```python
from build123d import *

# Parameters (mm, degrees)
SKETCH1_W            = 58.2
SKETCH1_H            = 40
BOSS_EXTRUDE1_DEPTH  = 27
SKETCH2_R            = 3
BOSS_EXTRUDE2_DEPTH  = 2
SKETCH3_R            = 2
CUT_EXTRUDE1_DEPTH   = 31
SKETCH4_R            = 3
BOSS_EXTRUDE3_DEPTH  = 2
SKETCH5_R            = 2
CUT_EXTRUDE2_DEPTH   = 31
SKETCH6_R            = 3
BOSS_EXTRUDE4_DEPTH  = 2
SKETCH7_R            = 2
CUT_EXTRUDE3_DEPTH   = 31
SKETCH8_R            = 3
BOSS_EXTRUDE5_DEPTH  = 2
SKETCH9_R            = 2
CUT_EXTRUDE4_DEPTH   = 31
SKETCH10_R           = 8
BOSS_EXTRUDE6_DEPTH  = 4.5
SKETCH11_R           = 4
CUT_EXTRUDE5_DEPTH   = 36
BOSS_EXTRUDE7_START  = 2
SKETCH12_R           = 3
BOSS_EXTRUDE7_DEPTH  = 2
BOSS_EXTRUDE8_START  = 2
SKETCH13_R           = 3
BOSS_EXTRUDE8_DEPTH  = 2
BOSS_EXTRUDE9_START  = 4.5
SKETCH15_R           = 8
BOSS_EXTRUDE9_DEPTH  = 4.5
SKETCH18_R           = 2
CUT_EXTRUDE11_DEPTH  = 78.32716211
SKETCH19_R           = 4
CUT_EXTRUDE12_DEPTH  = 78.32716211
SKETCH20_R           = 2
CUT_EXTRUDE13_DEPTH  = 78.32716211
SKETCH24_R           = 3
BOSS_EXTRUDE11_DEPTH = 2
SKETCH25_R           = 3
BOSS_EXTRUDE12_DEPTH = 2
BOSS_EXTRUDE13_START = 2
SKETCH26_R           = 3
BOSS_EXTRUDE13_DEPTH = 2
BOSS_EXTRUDE14_START = 2
SKETCH27_R           = 3
BOSS_EXTRUDE14_DEPTH = 2
FILLET5_R            = 1.5
FILLET6_R            = 1.5


with BuildPart() as part:
    # Sketch1 → Boss-Extrude1 (new body)
    with BuildSketch(Plane(origin=(0, 0, 0), x_dir=(1, 0, 0), z_dir=(0, 1, 0))):
        with Locations((-29.1, 20)):
            Rectangle(SKETCH1_W, SKETCH1_H)
    extrude(amount=BOSS_EXTRUDE1_DEPTH)

    # Sketch2 → Boss-Extrude2 (add)
    with BuildSketch(Plane(origin=(0, 27, 0), x_dir=(1, 0, 0), z_dir=(0, 1, 0))):
        with Locations(Location((-49.1, 34, 0), (0, 0, 270))):
            Circle(SKETCH2_R)
    extrude(amount=BOSS_EXTRUDE2_DEPTH)

    # Sketch3 → Cut-Extrude1 (cut)
    with BuildSketch(Plane(origin=(0, 29, 0), x_dir=(1, 0, 0), z_dir=(0, 1, 0))):
        with Locations(Location((-49.1, 34, 0), (0, 0, 270))):
            Circle(SKETCH3_R)
    extrude(amount=-CUT_EXTRUDE1_DEPTH, mode=Mode.SUBTRACT)

    # Sketch4 → Boss-Extrude3 (add)
    with BuildSketch(Plane(origin=(0, 27, 0), x_dir=(1, 0, 0), z_dir=(0, 1, 0))):
        with Locations(Location((-9.1, 34, 0), (0, 0, 270))):
            Circle(SKETCH4_R)
    extrude(amount=BOSS_EXTRUDE3_DEPTH)

    # Sketch5 → Cut-Extrude2 (cut)
    with BuildSketch(Plane(origin=(0, 29, 0), x_dir=(1, 0, 0), z_dir=(0, 1, 0))):
        with Locations(Location((-9.1, 34, 0), (0, 0, 270))):
            Circle(SKETCH5_R)
    extrude(amount=-CUT_EXTRUDE2_DEPTH, mode=Mode.SUBTRACT)

    # Sketch6 → Boss-Extrude4 (add)
    with BuildSketch(Plane(origin=(0, 27, 0), x_dir=(1, 0, 0), z_dir=(0, 1, 0))):
        with Locations(Location((-49.1, 6, 0), (0, 0, 270))):
            Circle(SKETCH6_R)
    extrude(amount=BOSS_EXTRUDE4_DEPTH)

    # Sketch7 → Cut-Extrude3 (cut)
    with BuildSketch(Plane(origin=(0, 29, 0), x_dir=(1, 0, 0), z_dir=(0, 1, 0))):
        with Locations(Location((-49.1, 6, 0), (0, 0, 270))):
            Circle(SKETCH7_R)
    extrude(amount=-CUT_EXTRUDE3_DEPTH, mode=Mode.SUBTRACT)

    # Sketch8 → Boss-Extrude5 (add)
    with BuildSketch(Plane(origin=(0, 27, 0), x_dir=(1, 0, 0), z_dir=(0, 1, 0))):
        with Locations(Location((-9.1, 6, 0), (0, 0, 270))):
            Circle(SKETCH8_R)
    extrude(amount=BOSS_EXTRUDE5_DEPTH)

    # Sketch9 → Cut-Extrude4 (cut)
    with BuildSketch(Plane(origin=(0, 29, 0), x_dir=(1, 0, 0), z_dir=(0, 1, 0))):
        with Locations(Location((-9.1, 6, 0), (0, 0, 270))):
            Circle(SKETCH9_R)
    extrude(amount=-CUT_EXTRUDE4_DEPTH, mode=Mode.SUBTRACT)

    # Sketch10 → Boss-Extrude6 (add)
    with BuildSketch(Plane(origin=(0, 27, 0), x_dir=(1, 0, 0), z_dir=(0, 1, 0))):
        with Locations(Location((-20.5, 20, 0), (0, 0, 270))):
            Circle(SKETCH10_R)
    extrude(amount=BOSS_EXTRUDE6_DEPTH)

    # Sketch11 → Cut-Extrude5 (cut)
    with BuildSketch(Plane(origin=(0, 31.5, 0), x_dir=(1, 0, 0), z_dir=(0, 1, 0))):
        with Locations(Location((-20.5, 20, 0), (0, 0, 270))):
            Circle(SKETCH11_R)
    extrude(amount=-CUT_EXTRUDE5_DEPTH, mode=Mode.SUBTRACT)

    # Sketch12 → Boss-Extrude7 (add)
    with BuildSketch(Plane.XZ.offset(BOSS_EXTRUDE7_START)):
        with Locations(Location((-49.1, -6, 0), (0, 0, 90))):
            Circle(SKETCH12_R)
    extrude(amount=-BOSS_EXTRUDE7_DEPTH)

    # Sketch13 → Boss-Extrude8 (add)
    with BuildSketch(Plane.XZ.offset(BOSS_EXTRUDE8_START)):
        with Locations(Location((-49.1, -34, 0), (0, 0, 90))):
            Circle(SKETCH13_R)
        with Locations(Location((-9.1, -6, 0), (0, 0, 90))):
            Circle(SKETCH13_R)
        with Locations(Location((-9.1, -34, 0), (0, 0, 90))):
            Circle(SKETCH13_R)
    extrude(amount=-BOSS_EXTRUDE8_DEPTH)

    # Sketch15 → Boss-Extrude9 (add)
    with BuildSketch(Plane.XZ.offset(BOSS_EXTRUDE9_START)):
        with Locations(Location((-20.5, -20, 0), (0, 0, 90))):
            Circle(SKETCH15_R)
    extrude(amount=-BOSS_EXTRUDE9_DEPTH)

    # Sketch18 → Cut-Extrude11 (cut, through all)
    with BuildSketch(Plane(origin=(0, 0, 0), x_dir=(1, 0, 0), z_dir=(0, 1, 0))):
        with Locations(Location((-9.1, 6, 0), (0, 0, 270))):
            Circle(SKETCH18_R)
    extrude(amount=-CUT_EXTRUDE11_DEPTH, mode=Mode.SUBTRACT)

    # Sketch19 → Cut-Extrude12 (cut, through all)
    with BuildSketch(Plane(origin=(0, 0, 0), x_dir=(1, 0, 0), z_dir=(0, 1, 0))):
        with Locations(Location((-20.5, 20, 0), (0, 0, 270))):
            Circle(SKETCH19_R)
    extrude(amount=-CUT_EXTRUDE12_DEPTH, mode=Mode.SUBTRACT)

    # Sketch20 → Cut-Extrude13 (cut, through all)
    with BuildSketch(Plane(origin=(0, 0, 0), x_dir=(1, 0, 0), z_dir=(0, 1, 0))):
        with Locations(Location((-49.1, 34, 0), (0, 0, 270))):
            Circle(SKETCH20_R)
        with Locations(Location((-49.1, 6, 0), (0, 0, 270))):
            Circle(SKETCH20_R)
        with Locations(Location((-9.1, 34, 0), (0, 0, 270))):
            Circle(SKETCH20_R)
    extrude(amount=-CUT_EXTRUDE13_DEPTH, mode=Mode.SUBTRACT)

    # Sketch24 → Boss-Extrude11 (add)
    with BuildSketch(Plane(origin=(0, 27, 0), x_dir=(1, 0, 0), z_dir=(0, 1, 0))):
        with Locations(Location((-36.2, 15, 0), (0, 0, 270))):
            Circle(SKETCH24_R)
    extrude(amount=BOSS_EXTRUDE11_DEPTH)

    # Sketch25 → Boss-Extrude12 (add)
    with BuildSketch(Plane(origin=(0, 27, 0), x_dir=(1, 0, 0), z_dir=(0, 1, 0))):
        with Locations(Location((-36.2, 25, 0), (0, 0, 270))):
            Circle(SKETCH25_R)
    extrude(amount=BOSS_EXTRUDE12_DEPTH)

    # Sketch26 → Boss-Extrude13 (add)
    with BuildSketch(Plane.XZ.offset(BOSS_EXTRUDE13_START)):
        with Locations(Location((-36.2, -15, 0), (0, 0, 90))):
            Circle(SKETCH26_R)
    extrude(amount=-BOSS_EXTRUDE13_DEPTH)

    # Sketch27 → Boss-Extrude14 (add)
    with BuildSketch(Plane.XZ.offset(BOSS_EXTRUDE14_START)):
        with Locations(Location((-36.2, -25, 0), (0, 0, 90))):
            Circle(SKETCH27_R)
    extrude(amount=-BOSS_EXTRUDE14_DEPTH)

    # Fillet5
    fillet5_edges = [part.edges().sort_by_distance(p)[0] for p in [
        (-58.2, 27, -20),
        (-29.1, 27, 0),
        (0, 27, -20),
        (-29.1, 0, 0),
        (-58.2, 0, -20),
        (-29.1, 0, -40),
        (0, 0, -20),
        (0, 13.5, 0),
        (-58.2, 13.5, 0),
        (-58.2, 13.5, -40),
        (-29.1, 27, -40),
    ]]
    fillet(fillet5_edges, radius=FILLET5_R)

    # Fillet6
    # the kernel refuses this fillet: 1.5 mm, written as the material it takes off along each edge
    with BuildSketch(Plane(origin=(-1.5, 1.5, -38.5), x_dir=(0, 0, -1), z_dir=(1, 0, 0))) as fillet6_piece_1_section:
        Polygon((0, 0), (FILLET6_R, 0), (FILLET6_R, -FILLET6_R), (0, -FILLET6_R), align=None)
    fillet6_piece_1 = extrude(amount=FILLET6_R, mode=Mode.PRIVATE)
    fillet6_piece_1 = fillet6_piece_1 - Plane(origin=(-1.5, 1.5, -38.5), x_dir=(0, 0.7071067811865475, 0.7071067811865475), z_dir=(1, 0, 0)) * Sphere(FILLET6_R, mode=Mode.PRIVATE)
    add(fillet6_piece_1, mode=Mode.SUBTRACT)
    with BuildSketch(Plane(origin=(-1.5, 25.5, -38.5), x_dir=(0, 0, -1), z_dir=(1, 0, 0))) as fillet6_piece_2_section:
        Polygon((0, 0), (FILLET6_R, 0), (FILLET6_R, FILLET6_R), (0, FILLET6_R), align=None)
    fillet6_piece_2 = extrude(amount=FILLET6_R, mode=Mode.PRIVATE)
    fillet6_piece_2 = fillet6_piece_2 - Plane(origin=(-1.5, 25.5, -38.5), x_dir=(0, -0.7071067811865475, 0.7071067811865475), z_dir=(1, 0, 0)) * Sphere(FILLET6_R, mode=Mode.PRIVATE)
    add(fillet6_piece_2, mode=Mode.SUBTRACT)
    with BuildSketch(Plane(origin=(0, 1.5, -40), x_dir=(0, 0, 1), z_dir=(0, 1, 0))) as fillet6_piece_3:
        with BuildLine():
            CenterArc((FILLET6_R, -FILLET6_R), FILLET6_R, 90, 90)
            Line((0, -FILLET6_R), (0, 0))
            Line((0, 0), (FILLET6_R, 0))
        make_face()
    extrude(amount=24, mode=Mode.SUBTRACT)


solid = part.part
```
Source: CAD feature listing. Evaluate the final solid. Frame: model axes, mm. A direction names the side the tool comes from. Round coordinates to 2 decimals unless told otherwise and drop trailing zeros. Loops run counter-clockwise (first coordinate to the right, second up) from the corner with the lowest first, then second, coordinate; pieces in that order, holes last.
1. Mould query, pull axis Z, two halves, no side actions, for faces 1 (the flat face through (-48, -2, -32)), 2 (the cylindrical face through (-49, -1, -37)), 3 (the cylindrical face through (-46.438, -1.014, -4.616)), 4 (the cylindrical face through (-57.77, 13.67, -0.45)). Classes: released by +Z, released by -Z, zero draft, split by the parting line, or undercut.
2. Section query C-C on x = -20.5. Output: boundary loops of the cut face in (y, z), and give its area (3 significant figures).
3. Section query D-D on y = 19.5. Output: boundary loops of the cut face in (x, z), and give its area (3 significant figures).
4. Contact query for flat-ended pins moving along their axis: pin 1 (5 mm diameter, centred on x = -35.5, z = -16, fed in from +Y); pin 2 (5 mm diameter, centred on x = -47.5, z = -34, fed in from -Y); pin 3 (2 mm diameter, centred on x = -7, z = -17.5, fed in from +Y). Output: stop coordinate, or through.
5. Ray query, L1, parallel to Z at x = -49, y = 13; L2, parallel to X at y = 11.5, z = -34; L3, parallel to X at y = 18, z = -20. Return the intervals inside material, ascending.
6. Access query for faces 5 (the cylindrical face through (-38.23, -1.01, -27.21)), 6 (the flat face through (-36, -2, -25)), 7 (the cylindrical face through (-8.2, 27.99, -3.14)). Directions: +Z, -Z, +X, -X, +Y, -Y. A direction counts if a zero-diameter tool reaches every point of the face in a straight line with its end or side. Return the directions, or none.
7. Section query A-A on z = -6. Give the number of separate pieces and of enclosed holes in the cut face, and give its area (3 significant figures).
Answers below:
1. face 1: zero draft
1. face 2: undercut
1. face 3: undercut
1. face 4: released by +Z
2. outline: (-4.5, -28) - (0, -28) - (0, -38.5) arc R1.5 ccw to (1.5, -40) - (25.5, -40) arc R1.5 ccw to (27, -38.5) - (27, -28) - (31.5, -28) - (31.5, -24) - (-4.5, -24) - close; (-4.5, -16) - (31.5, -16) - (31.5, -12) - (27, -12) - (27, -1.5) arc R1.5 ccw to (25.5, 0) - (1.5, 0) arc R1.5 ccw to (0, -1.5) - (0, -12) - (-4.5, -12) - close
2. area: 934 mm2
3. outline: (-58.2, -38.5) arc R1.5 ccw to (-56.7, -40) - (-1.5, -40) arc R1.5 ccw to (0, -38.5) - (0, -1.5) arc R1.5 ccw to (-1.5, 0) - (-56.7, 0) arc R1.5 ccw to (-58.2, -1.5) - close; hole circle Ø4 at (-49.1, -34); hole circle Ø4 at (-49.1, -6); hole circle Ø8 at (-20.5, -20); hole circle Ø4 at (-9.1, -34); hole circle Ø4 at (-9.1, -6)
3. area: 2,230 mm2
4. pin 1: stops at y = 29
4. pin 2: stops at y = -2
4. pin 3: stops at y = 27
5. L1: z = -40 to -36, -32 to -8, -4 to 0
5. L2: x = -58.2 to -51.1, -47.1 to -11.1, -7.1 to 0
5. L3: x = -58.2 to -24.5, -16.5 to 0
6. face 5: -Y
6. face 6: +Z, -Z, -X, -Y
6. face 7: +Y
7. separate pieces: 3
7. enclosed holes: 0
7. area: 1,370 mm2
